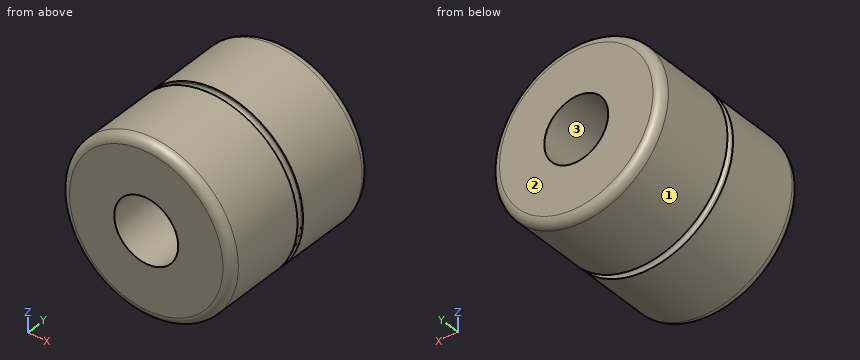
```python
from build123d import *

# Parameters (mm, degrees)
F0_R     = 12.7
F0_R_2   = 4.7625
F1_DEPTH = 12.7
F3_R     = 1.27
F6_R     = 0.6168431606


with BuildPart() as f1:
    # F0 (on Front) → F1 (new body, symmetric)
    with BuildSketch(Plane.XZ):
        Circle(F0_R)
        Circle(F0_R_2, mode=Mode.SUBTRACT)
    extrude(amount=F1_DEPTH, both=True)

    # F3
    f3_edges = [f1.edges().sort_by_distance(p)[0] for p in [
        (-12.7, 12.7, 0),
        (-12.7, -12.7, 0),
    ]]
    fillet(f3_edges, radius=F3_R)

    # F7: sweep along a path in F4
    with BuildLine(Plane(origin=(0, 0, 0), x_dir=(-1, 0, 0), z_dir=(0, 1, 0))) as f7_path:
        CenterArc((0, 0), 12.319, 0, 360)
    # F6 (on line) → F7 (sweep, cut)
    with BuildSketch(Plane.YZ):
        with Locations((0, 12.3572489247)):
            Circle(F6_R)
    sweep(path=f7_path.line, mode=Mode.SUBTRACT)


solid = f1.part
```
Check sheet for the modelled part. Datum: model origin and axes. Units: mm. Face numbers are marked on the shaded views. Coordinates: 2 decimals unless noted, no trailing zeros. Loops run counter-clockwise (first coordinate to the right, second up) from the corner with the lowest first, then second, coordinate; pieces in that order, holes last.
1) Sectioned sample at A-A (x = 0). Record the boundary of the cut face in (y, z), and give its area (3 significant figures).
2) Material ranges on probe 1 along Z at (x, y) = (0, 2.5); probe 2 along Z at (x, y) = (-4.25, 7.5); probe 3 along X at (y, z) = (10, 3), recorded low to high.
3) Sectioned sample at C-C (y = 6.5). Record the boundary of the cut face in (x, z) (1 decimal), and give its area (3 significant figures).
4) Gauge pin test, flat ends, axial feed: pin 1 (6 mm diameter, centred on x = 4.5, y = 6.5, fed in from +Z); pin 2 (2 mm diameter, centred on x = -10, y = -9.5, fed in from +Z); pin 3 (6 mm diameter, centred on x = -5.5, y = -2, fed in from -Z). Record the tip position at first contact, or that the pin passes through.
5) Release check for a two-part mould opening along X. For the marked faces 1, 2 and 3 record: released by +X, released by -X, zero draft, split by the parting line, or undercut.
6) Sectioned sample at B-B (z = 0). Record the boundary of the cut face in (x, y), and give its area (3 significant figures).
Check sheet entries:
1. outline: (-12.7, -11.43) arc R1.27 ccw to (-11.43, -12.7) - (-0.51, -12.7) arc R0.62 cw (long way) to (0.51, -12.7) - (11.43, -12.7) arc R1.27 ccw to (12.7, -11.43) - (12.7, -4.76) - (-12.7, -4.76) - close; (-12.7, 4.76) - (12.7, 4.76) - (12.7, 11.43) arc R1.27 ccw to (11.43, 12.7) - (0.51, 12.7) arc R0.62 cw (long way) to (-0.51, 12.7) - (-11.43, 12.7) arc R1.27 ccw to (-12.7, 11.43) - close
1. area: 400 mm2
2. probe 1: z = -12.7 to -4.76, 4.76 to 12.7
2. probe 2: z = -11.97 to -2.15, 2.15 to 11.97
2. probe 3: x = -12.34 to -3.7, 3.7 to 12.34
3. outline: circle Ø25.4 at (0, 0); hole circle Ø9.5 at (0, 0)
3. area: 435 mm2
4. pin 1: stops at z = 12.61
4. pin 2: stops at z = 8.96
4. pin 3: stops at z = -12.45
5. face 1: split by the parting line
5. face 2: zero draft
5. face 3: undercut
6. outline: (-12.7, -11.43) arc R1.27 ccw to (-11.43, -12.7) - (-4.76, -12.7) - (-4.76, 12.7) - (-11.43, 12.7) arc R1.27 ccw to (-12.7, 11.43) - (-12.7, 0.51) arc R0.62 cw (long way) to (-12.7, -0.51) - close; (4.76, -12.7) - (11.43, -12.7) arc R1.27 ccw to (12.7, -11.43) - (12.7, -0.51) arc R0.62 cw (long way) to (12.7, 0.51) - (12.7, 11.43) arc R1.27 ccw to (11.43, 12.7) - (4.76, 12.7) - close
6. area: 400 mm2
